```python
from build123d import *

# Parameters (mm, degrees)
SKETCH1_W                                       = 152.4
SKETCH1_H                                       = 101.6
BOSS_EXTRUDE1_DEPTH                             = 2.54
FILLET1_R                                       = 1.5875
CSK_FOR_M3_FLAT_HEAD_MACHINE_SCREW1_D           = 3.4
CSK_FOR_M3_FLAT_HEAD_MACHINE_SCREW1_DEPTH       = 6.35
CSK_FOR_M3_FLAT_HEAD_MACHINE_SCREW1_CSINK_D     = 6.3
CSK_FOR_M3_FLAT_HEAD_MACHINE_SCREW1_CSINK_ANGLE = 90
CSK_FOR_M3_FLAT_HEAD_MACHINE_SCREW1_TIP         = 1.021463052


with BuildPart() as part:
    # Sketch1 → Boss-Extrude1 (new body)
    with BuildSketch(Plane.XY):
        with Locations((76.2, 50.8)):
            Rectangle(SKETCH1_W, SKETCH1_H)
    extrude(amount=BOSS_EXTRUDE1_DEPTH)

    # Fillet1
    fillet1_edges = [part.edges().sort_by_distance(p)[0] for p in [
        (152.4, 50.8, 2.54),
        (76.2, 101.6, 2.54),
        (0, 50.8, 2.54),
        (76.2, 0, 2.54),
    ]]
    fillet(fillet1_edges, radius=FILLET1_R)

    # CSK for M3 Flat Head Machine Screw1
    with Locations(Plane.XY.offset(2.54)):
        with Locations((6.35, 95.25), (6.35, 6.35), (146.05, 6.35), (146.05, 95.25)):
            CounterSinkHole(CSK_FOR_M3_FLAT_HEAD_MACHINE_SCREW1_D / 2, CSK_FOR_M3_FLAT_HEAD_MACHINE_SCREW1_CSINK_D / 2, depth=CSK_FOR_M3_FLAT_HEAD_MACHINE_SCREW1_DEPTH, counter_sink_angle=CSK_FOR_M3_FLAT_HEAD_MACHINE_SCREW1_CSINK_ANGLE)
            with Locations((0, 0, -(CSK_FOR_M3_FLAT_HEAD_MACHINE_SCREW1_DEPTH + CSK_FOR_M3_FLAT_HEAD_MACHINE_SCREW1_TIP / 2))):  # 118° drill point
                Cone(0, CSK_FOR_M3_FLAT_HEAD_MACHINE_SCREW1_D / 2, CSK_FOR_M3_FLAT_HEAD_MACHINE_SCREW1_TIP, mode=Mode.SUBTRACT)


solid = part.part
```
Verification items for the finished model (mm, model axes). Round coordinates to 2 decimals unless told otherwise and drop trailing zeros. Write each loop counter-clockwise with the first axis right and the second up, starting at its lowest first coordinate (ties: lowest second). Pieces come first, ordered by that corner, then holes.
1. Draft check along Y on faces 1 (the cylindrical face through (6.571, 8.036, 0.537)), 2 (the flat face through (75, 51, 2.54)). Enter one of: +Y half, -Y half, draft (parallel to the pull), parting line (faces both ways), or undercut.
2. Section check C-C on z = 2.1. Enter the section's corners in (x, y), plus the area to 3 significant figures.
3. Section check A-A on y = 95.25. State how many separate pieces and enclosed holes the cut face has, plus the area to 3 significant figures.
4. Scan lines: L1, parallel to Y at x = 146.05, z = 0.5; L2, parallel to X at y = 95.25, z = 0.65; L3, parallel to X at y = 96.5, z = 2.4. Record each from-to range of solid material in increasing order.
5. Gauge pin test, flat ends, axial feed: P1, Ø4.5, axis at x = 146.05, y = 6.35, coming from the +Z side; P2, Ø2, axis at x = 6.35, y = 95.25, coming from the +Z side; P3, Ø1, axis at x = 35.5, z = 2, coming from the -Y side; P4, Ø1.5, axis at x = 100, z = 2, coming from the -Y side. Record the tip position at first contact, or that the pin passes through.
Answer:
1. face 1: undercut
1. face 2: draft
2. outline: (0.49, 0.49) - (151.91, 0.49) - (151.91, 101.11) - (0.49, 101.11) - close; hole circle Ø5.42 at (6.35, 6.35); hole circle Ø5.42 at (6.35, 95.25); hole circle Ø5.42 at (146.05, 6.35); hole circle Ø5.42 at (146.05, 95.25)
2. area: 15,100 mm2
3. separate pieces: 3
3. enclosed holes: 0
3. area: 365 mm2
4. L1: y = 0 to 4.65, 8.05 to 93.55, 96.95 to 101.6
4. L2: x = 0 to 4.65, 8.05 to 144.35, 147.75 to 152.4
4. L3: x = 0.94 to 3.61, 9.09 to 143.31, 148.79 to 151.46
5. P1: stops at z = 1.64
5. P2: passes through
5. P3: stops at y = 0.1
5. P4: stops at y = 0.03
